Could you check a few things on this model? Use its own coordinates, in mm. Face numbers are marked on the shaded views. A direction names the side the tool comes from. Coordinates: 2 decimals unless noted, no trailing zeros. Loops run counter-clockwise (first coordinate to the right, second up) from the corner with the lowest first, then second, coordinate; pieces in that order, holes last.
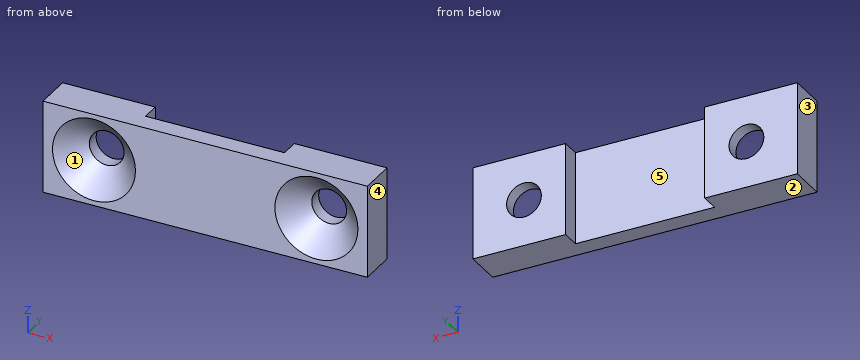
Autodesk Fusion 360 part; units mm, degrees
sketch "Sketch1" plane through (0, 0, 0) normal (0, 1, 0) x (1, 0, 0)
  line L0 (-17.5, 5) -> (17.5, 5)
  line L1 (17.5, 5) -> (17.5, -5)
  line L2 (17.5, -5) -> (-17.5, -5)
  line L3 (-17.5, -5) -> (-17.5, 5)
  line L4 (-17.5, 5) -> (17.5, -5) construction
  line L5 (17.5, 5) -> (-17.5, -5) construction
  line L6 (-7.5, 5) -> (7.5, 5)
  line L7 (7.5, 5) -> (7.5, -5)
  line L8 (7.5, -5) -> (-7.5, -5)
  line L9 (-7.5, -5) -> (-7.5, 5)
  line L10 (-7.5, 5) -> (7.5, -5) construction
  line L11 (7.5, 5) -> (-7.5, -5) construction
  circle A0 centre (-12, 0) radius 1.875
  line L12 (0, -5) -> (0, -10.3309) construction
  line L13 (0, -5) -> (0, -10.3309) construction
  circle A1 centre (12, 0) radius 1.875
  dimension "d1" = 15
  dimension "d2" = 35
  dimension "d3" = 10
  dimension "d4" = 3.75
extrude "Extrude1" add sketch "Sketch1" along normal blind 2 contours L0 L2 L3 L9 | L0 L1 L2 L7 makes body 1 at (-16.2917, 0, 0) makes body 2 at (16.2917, 0, 0)
extrude "Extrude2" add sketch "Sketch1" against normal blind 2 bodies 1 2
chamfer "Chamfer1" distance 2.6 angle 45 2 edges at (-13.7481, -2, 0.678) (10.2519, -2, 0.678) on bodies 1
equation "d2 = 15 mm + 4 mm + 4 mm + 8 mm + 4 mm"
(1) Imagine slicing it at A-A, the plane y = 1.65. Write out the boundary of the cut face in (x, z) (3 decimals).
Answers:
outline: (-17.5, -5) - (-7.5, -5) - (-7.5, 5) - (-17.5, 5) - close; (7.5, -5) - (17.5, -5) - (17.5, 5) - (7.5, 5) - close; hole circle Ø3.75 at (-12, 0); hole circle Ø3.75 at (12, 0)
(2) I need wall thicknesses on probe 1 along X at (y, z) = (1.45, 0) (3 decimals); probe 2 along X at (y, z) = (1.1, -3.25); probe 3 along Z at (x, y) = (12, 1.35) (3 decimals). Which ranges of each line are inside material? Lowest first, please.
Answers:
probe 1: x = -17.5 to -13.875, -10.125 to -7.5, 7.5 to 10.125, 13.875 to 17.5
probe 2: x = -17.5 to -7.5, 7.5 to 17.5
probe 3: z = -5 to -1.875, 1.875 to 5
(3) Imagine slicing it at B-B, the plane x = -12. Write out the boundary of the cut face in (y, z) (3 decimals).
Answers:
outline: (-2, -5) - (2, -5) - (2, -1.875) - (0.6, -1.875) - (-2, -4.475) - close; (-2, 4.475) - (0.6, 1.875) - (2, 1.875) - (2, 5) - (-2, 5) - close
(4) Imagine slicing it at C-C, the plane z = 0. State how many separate pieces and enclosed holes the cut face has, and give its area (3 significant figures).
Answers:
separate pieces: 3
enclosed holes: 0
area: 66.5 mm2
(5) For pin 1 (5 mm diameter, centred on x = 12, z = 0, fed in from -Y) (3 decimals); pin 2 (2 mm diameter, centred on x = -12, z = 0, fed in from +Y); pin 3 (6 mm diameter, centred on x = 3.5, z = 1.5, fed in from +Y), each with a flat end and sliding along its axis, tell me the tip position at first contact or that it passes through.
Answers:
pin 1: stops at y = -0.025
pin 2: passes through
pin 3: stops at y = 0
(6) Imagine slicing it at D-D, the plane x = -5.5. Write out the boundary of the cut face in (y, z).
Answers:
outline: (-2, -5) - (0, -5) - (0, 5) - (-2, 5) - close
(7) Which directions (+Z, -Z, +X, -X, +Y, -Y) give clear straight access to the entire face, cutting with the end or side of a thin tool? Please do the marked faces 4 and 5.
Answers:
face 4: +Z, -Z, +X, +Y, -Y
face 5: +Z, -Z, +Y
(8) We'd pull the mould along Z, two halves only. Please class the marked faces 1, 2 and 3: +Z half, -Z half, draft (parallel to the pull), parting line (faces both ways), or undercut.
Answers:
face 1: undercut
face 2: -Z half
face 3: draft
